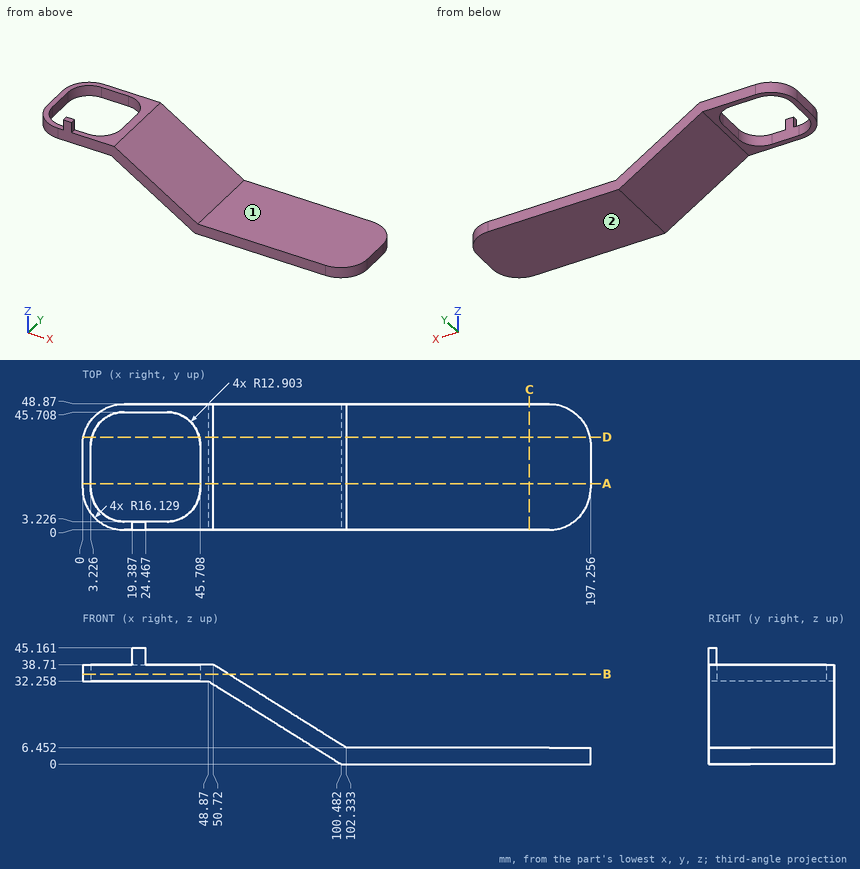
Geometry check sheet. Reference: drawing and pictorial views, mm from the part's lowest x, y, z. A direction names the side the tool comes from. Round coordinates to 2 decimals unless told otherwise and drop trailing zeros. Loops run counter-clockwise (first coordinate to the right, second up) from the corner with the lowest first, then second, coordinate; pieces in that order, holes last. Notation, with made-up numbers: (28.5, 67) - (69.5, 67) arc R22 cw to (69.5, 89) - close; hole circle Ø1 at (-4.75, 64). An arc over 180 degrees is marked (long way). Answer in a Markdown table with one row per item. Add a question column.
Q1. Section check B-B on z = 35. Enter the section's corners in (x, y) (1 decimal).
Q2. Section check D-D on y = 36. Enter the section's corners in (x, z), plus the area to 3 significant figures.
Q3. Tool access check on the marked faces 1 and 2. Record the directions out of +Z, -Z, +X, -X, +Y, -Y that give a thin tool (end or side, any length) a straight path to the whole face; none if there is none.
Q4. Section check A-A on y = 18. Enter the section's corners in (x, z) (1 decimal).
Q5. Section check C-C on x = 173.5. Enter the section's corners in (y, z).
Q6. Gauge pin test, flat ends, axial feed: pin 1 (10.5 mm diameter, centred on x = 27.5, z = 40, fed in from +Y); pin 2 (8 mm diameter, centred on y = 30, z = 28.5, fed in from +X) (1 decimal); pin 3 (10 mm diameter, centred on y = 15, z = 27.5, fed in from +X) (1 decimal); pin 4 (2.5 mm diameter, centred on y = 2, z = 43.5, fed in from -X). Record the tip position at first contact, or that the pin passes through.
Q7. Material ranges on line 1 (Z direction, x = 186.5, y = 28.5); line 2 (X direction, y = 24.5, z = 34.5) (1 decimal); line 3 (X direction, y = 7, z = 13.5) (1 decimal), recorded low to high.
Found:
| question | item | result |
|---|---|---|
| 1 | outline | (0, 16.1) arc R16.1 ccw to (16.1, 0) - (56.7, 0) - (56.7, 48.9) - (16.1, 48.9) arc R16.1 ccw to (0, 32.7) - close; hole (3.2, 16.1) arc R12.9 ccw to (16.1, 3.2) - (32.8, 3.2) arc R12.9 ccw to (45.7, 16.1) - (45.7, 32.8) arc R12.9 ccw to (32.8, 45.7) - (16.1, 45.7) arc R12.9 ccw to (3.2, 32.8) - close |
| 2 | outline | (0.33, 32.26) - (3.63, 32.26) - (3.63, 38.71) - (0.33, 38.71) - close; (45.31, 32.26) - (48.87, 32.26) - (100.48, 0) - (196.92, 0) - (196.92, 6.45) - (102.33, 6.45) - (50.72, 38.71) - (45.31, 38.71) - close |
| 2 | area | 1,060 mm² |
| 3 | face 1 | +Z, +X, +Y, -Y |
| 3 | face 2 | -Z, +X, -X, +Y, -Y |
| 4 | outline | (0, 32.3) - (3.2, 32.3) - (3.2, 38.7) - (0, 38.7) - close; (45.7, 32.3) - (48.9, 32.3) - (100.5, 0) - (197.3, 0) - (197.3, 6.5) - (102.3, 6.5) - (50.7, 38.7) - (45.7, 38.7) - close |
| 5 | outline | (0, 0) - (48.87, 0) - (48.87, 6.45) - (0, 6.45) - close |
| 6 | pin 1 | stops at y = 48.87 |
| 6 | pin 2 | stops at x = 73.5 |
| 6 | pin 3 | stops at x = 76.7 |
| 6 | pin 4 | stops at x = 19.39 |
| 7 | line 1 | z = 0 to 6.45 |
| 7 | line 2 | x = 0 to 3.2, 45.7 to 57.5 |
| 7 | line 3 | x = 78.9 to 91.1 |
